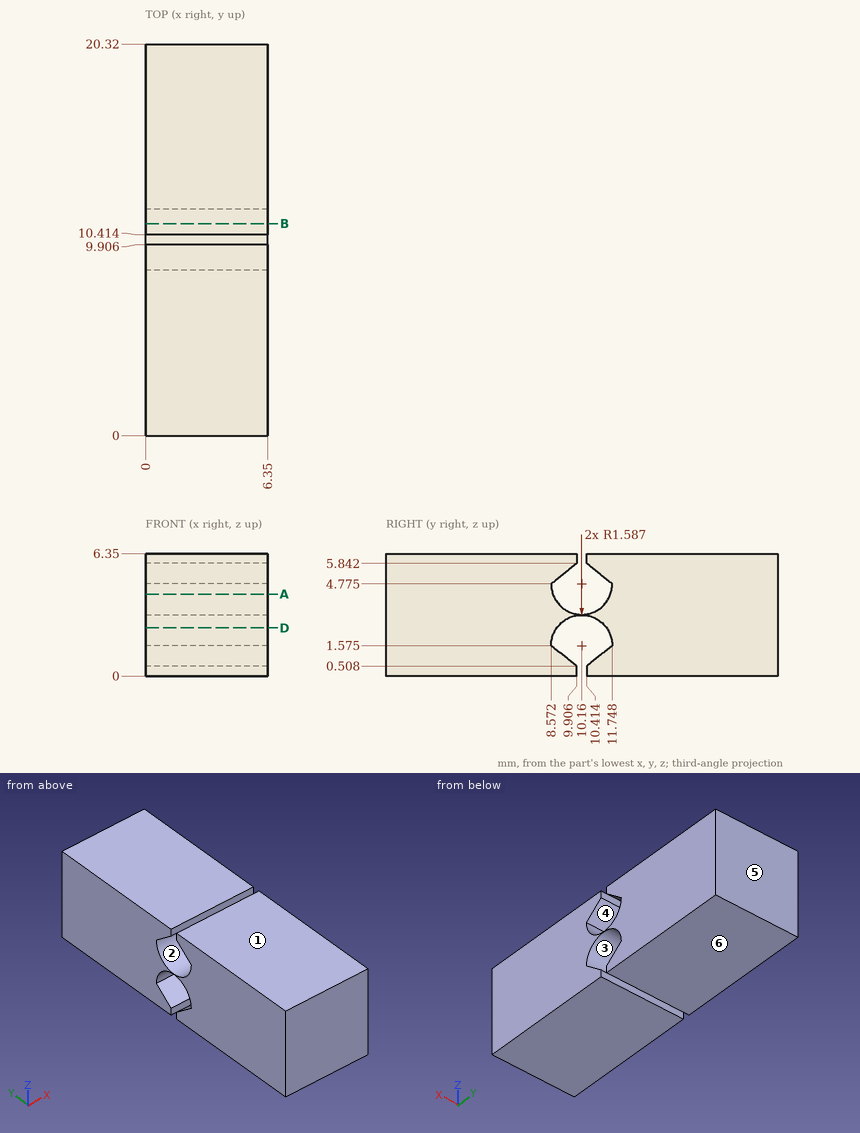
Study the drawing (mm; zero at the part's minimum x, y, z) and answer. A direction names the side the tool comes from. Coordinates: 2 decimals unless noted, no trailing zeros. Loops run counter-clockwise (first coordinate to the right, second up) from the corner with the lowest first, then second, coordinate; pieces in that order, holes last. Notation, with made-up numbers: M 23,28.25 L 66,28.25 A36 cw 66,64.25 Z; hole C -25.75,-22 d9. An arc over 180 degrees is marked long. Answer in a Markdown table with one row per item. Add a question column.
1. Find section A-A, the plane z = 4.25. Write down the section's boundary in (x, y), then the cut area to 3 significant figures.
2. The mould has two halves that part along Y. Classify the marked faces 3, 4, 5 and 6: pulls with the +Y half, pulls with the -Y half, needs draft (parallel to the pull), parting line crosses it, or undercut.
3. Find section D-D, the plane z = 2.5. Write down the section's boundary in (x, y).
4. Find section B-B, the plane y = 11. Write down the section's boundary in (x, z).
5. A flat-ended cylindrical pin translates along its axis: P1, Ø3, axis at y = 6.5, z = 4, coming from the -X side. Find the tip coordinate at first contact, or state that the pin passes through.
6. A tool of negligible diameter and unlimited length cuts with its end or side. For the marked faces 1 and 2, from which of +Z, -Z, +X, -X, +Y, -Y can it reach the whole face along a straight path? Write none if from no direction.
7. Consider L1, parallel to Y at x = 0.75, z = 4.75; L2, parallel to Y at x = 1.75, z = 4.25. Determine where each line is inside the solid, lowest interval first.
Reported:
| question | item | result |
|---|---|---|
| 1 | outline | M 0,0 L 6.35,0 L 6.35,8.66 L 0,8.66 Z; M 0,11.66 L 6.35,11.66 L 6.35,20.32 L 0,20.32 Z |
| 1 | area | 110 mm^2 |
| 2 | face 3 | undercut |
| 2 | face 4 | undercut |
| 2 | face 5 | pulls with the +Y half |
| 2 | face 6 | needs draft |
| 3 | outline | M 0,0 L 6.35,0 L 6.35,8.87 L 0,8.87 Z; M 0,11.45 L 6.35,11.45 L 6.35,20.32 L 0,20.32 Z |
| 4 | outline | M 0,0 L 6.35,0 L 6.35,0.98 L 0,0.98 Z; M 0,2.92 L 6.35,2.92 L 6.35,3.43 L 0,3.43 Z; M 0,5.37 L 6.35,5.37 L 6.35,6.35 L 0,6.35 Z |
| 5 | P1 | stops at x = 0 |
| 6 | face 1 | +Z, +X, -X, +Y, -Y |
| 6 | face 2 | +X, -X |
| 7 | L1 | y = 0 to 8.57, 11.75 to 20.32 |
| 7 | L2 | y = 0 to 8.66, 11.66 to 20.32 |
